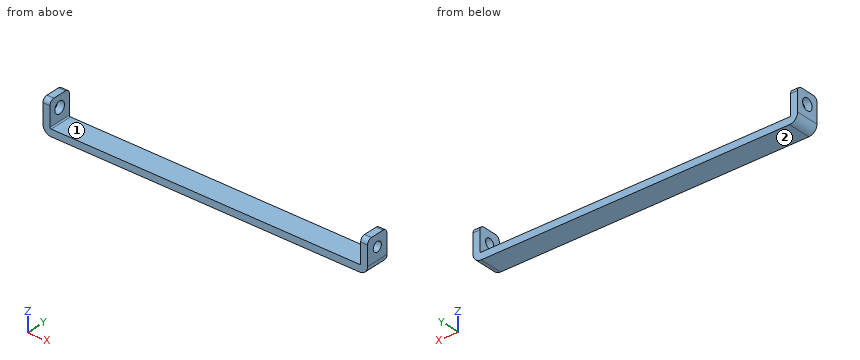
from build123d import *

# Parameters (mm, degrees)
SKETCH_1_R             = 2.5
SKETCH_1_R_2           = 2
SM_BASE_FLANGE_1_DEPTH = 3
OTHER_START            = 78.048031103
OTHER_1_OUTLINE_R      = 2.5
OTHER_1_OUTLINE_R_2    = 2
OTHER_1_DEPTH          = 3
OTHER_START_2          = -68.951968897
OTHER_1_2_OUTLINE_W    = 10
OTHER_1_2_OUTLINE_H    = 3
OTHER_1_2_DEPTH        = 10
OTHER_START_3          = 81.048031103
OTHER_1_3_OUTLINE_W    = 10
OTHER_1_3_OUTLINE_H    = 3
OTHER_1_3_DEPTH        = 10
OTHER_START_4          = -58.951968897
OTHER_1_4_OUTLINE_R    = 2.5
OTHER_1_4_DEPTH        = 3.5
OTHER_START_5          = 77.548031103
OTHER_1_5_OUTLINE_R    = 2.5
OTHER_1_5_DEPTH        = 3.5
OTHER_START_6          = 13
OTHER_1_6_DEPTH        = 12
HOLE_WIZARD_M5_1_D     = 4.2


with BuildPart() as part:
    # 基体-法兰1: sheet metal written as solids
    # Sketch 1 → 基体-法兰1 (new body)
    with BuildSketch(Plane.XY):
        with BuildLine():
            Line((-66.951968897, 24.322862815), (89.048031103, 24.322862815))
            ThreePointArc((89.048031103, 24.322862815), (90.462244666, 23.737076377), (91.048031103, 22.322862815))
            Line((91.048031103, 22.322862815), (91.048031103, 16.322862815))
            ThreePointArc((91.048031103, 16.322862815), (90.462244666, 14.908649252), (89.048031103, 14.322862815))
            Line((89.048031103, 14.322862815), (-66.951968897, 14.322862815))
            ThreePointArc((-66.951968897, 14.322862815), (-68.366182459, 14.908649252), (-68.951968897, 16.322862815))
            Line((-68.951968897, 16.322862815), (-68.951968897, 22.322862815))
            ThreePointArc((-68.951968897, 22.322862815), (-68.366182459, 23.737076377), (-66.951968897, 24.322862815))
        make_face()
        with Locations((-63.951968897, 19.322862815)):
            Circle(SKETCH_1_R, mode=Mode.SUBTRACT)
        with Locations((86.048031103, 19.322862815)):
            Circle(SKETCH_1_R_2, mode=Mode.SUBTRACT)
    extrude(amount=-SM_BASE_FLANGE_1_DEPTH)

    # Other 1 2 outline → Other 1 2 (cut)
    with BuildSketch(Plane.YZ.offset(OTHER_START_2)):
        with Locations((19.322862815, -1.5)):
            Rectangle(OTHER_1_2_OUTLINE_W, OTHER_1_2_OUTLINE_H)
    extrude(amount=OTHER_1_2_DEPTH, mode=Mode.SUBTRACT)

    # Other 1 3 outline → Other 1 3 (cut)
    with BuildSketch(Plane.YZ.offset(OTHER_START_3)):
        with Locations((19.322862815, -1.5)):
            Rectangle(OTHER_1_3_OUTLINE_W, OTHER_1_3_OUTLINE_H)
    extrude(amount=OTHER_1_3_DEPTH, mode=Mode.SUBTRACT)

    # Other 1 4 outline → Other 1 4 (add)
    with BuildSketch(Plane.YZ.offset(OTHER_START_4)):
        with BuildLine():
            Line((14.322862815, 0), (24.322862815, 0))
            Line((24.322862815, 0), (24.322862815, 8.858407346))
            ThreePointArc((24.322862815, 8.858407346), (23.737076378, 10.272620909), (22.322862815, 10.858407346))
            Line((22.322862815, 10.858407346), (16.322862815, 10.858407346))
            ThreePointArc((16.322862815, 10.858407346), (14.908649252, 10.272620909), (14.322862815, 8.858407346))
            Line((14.322862815, 8.858407346), (14.322862815, 0))
        make_face()
        with Locations((19.322862815, 5.858407346)):
            Circle(OTHER_1_4_OUTLINE_R, mode=Mode.SUBTRACT)
    extrude(amount=OTHER_1_4_DEPTH)



with BuildPart() as body_2:
    # Other 1: read off the stored shape, not the designer's step
    # Other 1 outline → Other 1 (new body)
    with BuildSketch(Plane.YZ.offset(OTHER_START)):
        with Locations((19.322862815, 5.858407346)):
            Circle(OTHER_1_OUTLINE_R)
        with Locations((19.322862815, 5.858407346)):
            Circle(OTHER_1_OUTLINE_R_2, mode=Mode.SUBTRACT)
    extrude(amount=OTHER_1_DEPTH)


with BuildPart() as part_1:
    add(part.part)

    add(body_2.part)  # Other 1 5 merges body 2
    # Other 1 5 outline → Other 1 5 (add)
    with BuildSketch(Plane.YZ.offset(OTHER_START_5)):
        with BuildLine():
            Line((14.322862815, 0), (24.322862815, 0))
            Line((24.322862815, 0), (24.322862815, 8.858407346))
            ThreePointArc((24.322862815, 8.858407346), (23.737076378, 10.272620909), (22.322862815, 10.858407346))
            Line((22.322862815, 10.858407346), (16.322862815, 10.858407346))
            ThreePointArc((16.322862815, 10.858407346), (14.908649252, 10.272620909), (14.322862815, 8.858407346))
            Line((14.322862815, 8.858407346), (14.322862815, 0))
        make_face()
        with Locations((19.322862815, 5.858407346)):
            Circle(OTHER_1_5_OUTLINE_R, mode=Mode.SUBTRACT)
    extrude(amount=OTHER_1_5_DEPTH)

    # Other 1 6 outline → Other 1 6 (cut)
    with BuildSketch(Plane(origin=(0, 0, 0), x_dir=(1, 0, 0), z_dir=(0, 1, 0)).offset(OTHER_START_6)):
        with BuildLine():
            Line((-55.951968897, -0.5), (-55.951968897, -10.858407346))
            Line((-55.951968897, -10.858407346), (-55.451968897, -10.858407346))
            Line((-55.451968897, -10.858407346), (-55.451968897, 0))
            ThreePointArc((-55.451968897, 0), (-55.805522288, -0.146446609), (-55.951968897, -0.5))
        make_face()
        with BuildLine():
            Line((77.548031103, -10.858407346), (78.048031103, -10.858407346))
            Line((78.048031103, -10.858407346), (78.048031103, -0.5))
            ThreePointArc((78.048031103, -0.5), (77.901584494, -0.146446609), (77.548031103, 0))
            Line((77.548031103, 0), (77.548031103, -10.858407346))
        make_face()
        with BuildLine():
            Line((81.048031103, 3), (77.548031103, 3))
            ThreePointArc((77.548031103, 3), (80.022904837, 1.974873734), (81.048031103, -0.5))
            Line((81.048031103, -0.5), (81.048031103, 3))
        make_face()
        with BuildLine():
            ThreePointArc((-58.951968897, -0.5), (-57.926842631, 1.974873734), (-55.451968897, 3))
            Line((-55.451968897, 3), (-58.951968897, 3))
            Line((-58.951968897, 3), (-58.951968897, -0.5))
        make_face()
    extrude(amount=OTHER_1_6_DEPTH, mode=Mode.SUBTRACT)

    # M5 螺纹孔1 (through all)
    with Locations(Plane(origin=(81.048031103, 0, 0), x_dir=(0, 0, -1), z_dir=(1, 0, 0))):
        with Locations((-5.858407346, 19.322862815)):
            Hole(HOLE_WIZARD_M5_1_D / 2)


solid = part_1.part
Design review of the part built by this model. Coordinates are the model's own, in mm. Face numbers are marked on the shaded views. Round coordinates to 2 decimals unless told otherwise and drop trailing zeros. Loops run counter-clockwise (first coordinate to the right, second up) from the corner with the lowest first, then second, coordinate; pieces in that order, holes last. Notation, with made-up numbers: (-37, -16) -> (19, -16) arc R4 cw to (19, -11) -> close; hole circle Ø2 at (50.5, -23). An arc over 180 degrees is marked (long way). Use one line per item in the form item = value. Start each with the question number.
Q1. For pin 1 Ø3 at (x, y) = (-25, 22) entering from +Z, flat-tipped, find the tip position at first contact; note if it passes through.
Q2. We need section A-A on x = -11. Give the boundary of the cut face in (y, z).
Q3. Draft analysis for pull direction X (two halves, no side actions). For the marked faces 1 and 2, state which applies: +X half, -X half, draft (parallel to the pull), parting line (faces both ways), or undercut.
Q4. Wall thickness on line 1 along X through (y, z) = (19.75, 9.25); line 2 along Z through (x, y) = (27, 16.5); line 3 along X through (y, z) = (21.5, 6.5): over which ranges is each line inside the solid? List them lowest first. Write a range as [from, to].
Calculated:
q1.pin_1 = 0
q2.outline = (14.32, -3) -> (24.32, -3) -> (24.32, 0) -> (14.32, 0) -> close
q3.face_1 = undercut
q3.face_2 = draft
q4.line_1 = [-58.95, -55.95], [78.05, 81.05]
q4.line_2 = [-3, 0]
q4.line_3 = [78.05, 81.05]
